Source: CAD feature listing. Evaluate the final solid. Frame: model axes, mm. Face numbers are marked on the shaded views. A direction names the side the tool comes from. Coordinates: 2 decimals unless noted, no trailing zeros. Write each loop counter-clockwise with the first axis right and the second up, starting at its lowest first coordinate (ties: lowest second). Pieces come first, ordered by that corner, then holes. Notation, with made-up numbers: (-28.75, 43) -> (5.25, 43) arc R22 ccw to (5.25, 62) -> close; hole circle Ø6 at (-7.5, 67). An arc over 180 degrees is marked (long way). Write item = value, one per line.
from build123d import *

# Parameters (mm, degrees)
SKETCH003_W  = 130
SKETCH003_H  = 30
PAD003_DEPTH = 150
SKETCH002_W  = 180
SKETCH002_H  = 65
PAD002_DEPTH = 145


with BuildPart() as body002:
    # Sketch003 → Pad003 (new body)
    with BuildSketch(Plane.XZ):
        with Locations((13.539826, -11.184382)):
            Rectangle(SKETCH003_W, SKETCH003_H)
    extrude(amount=PAD003_DEPTH)


with BuildPart() as body002_1:
    # Body002 placement: moved
    add(body002.part.moved(Location((0, 2, 0))))


with BuildPart() as cut:
    # Sketch002 → Pad002 (new body)
    with BuildSketch(Plane.XZ):
        Rectangle(SKETCH002_W, SKETCH002_H)
    extrude(amount=PAD002_DEPTH)

    # Cut: cut Body002
    add(body002_1.part, mode=Mode.SUBTRACT)


with BuildPart() as cut_1:
    # Cut placement: moved
    add(cut.part.moved(Location((0, 1, 0))))


solid = cut_1.part
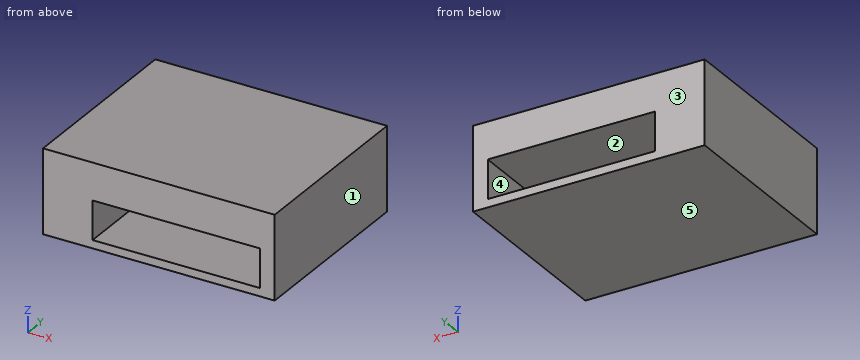
1) Cut plane C-C, the plane y = -60.5. Output: boundary loops of the cut face in (x, z).
Answer block:
outline = (-90, -32.5) -> (90, -32.5) -> (90, 32.5) -> (-90, 32.5) -> close; hole (-51.46, -26.18) -> (78.54, -26.18) -> (78.54, 3.82) -> (-51.46, 3.82) -> close
2) Cut plane A-A, the plane z = -4. Output: boundary loops of the cut face in (x, y), and give its area (3 significant figures).
Answer block:
outline = (-90, -144) -> (-51.46, -144) -> (-51.46, 1) -> (-90, 1) -> close; (78.54, -144) -> (90, -144) -> (90, 1) -> (78.54, 1) -> close
area = 7,250 mm2
3) Cut plane B-B, the plane x = -2. Output: boundary loops of the cut face in (y, z).
Answer block:
outline = (-144, -32.5) -> (1, -32.5) -> (1, -26.18) -> (-144, -26.18) -> close; (-144, 3.82) -> (1, 3.82) -> (1, 32.5) -> (-144, 32.5) -> close
4) Pull-direction query (Z, two-part tool) for the marked faces 3, 4 and 5; classes: +Z half, -Z half, draft (parallel to the pull), parting line (faces both ways), or undercut.
Answer block:
face_3 = draft
face_4 = undercut
face_5 = -Z half
5) First-contact query: pin 1 Ø12 at (x, z) = (-14.5, -25.5) entering from +Y. Flat tip, straight axial feed; report the tip coordinate or a pass-through.
Answer block:
pin_1 = 1
6) Material intervals for probe 1 along X at (y, z) = (-85.5, 1); probe 2 along Z at (x, y) = (-22, -97), sorted ascending. Write a range as [from, to].
Answer block:
probe_1 = [-90, -51.46], [78.54, 90]
probe_2 = [-32.5, -26.18], [3.82, 32.5]
7) Reachability of the marked faces 1 and 2 from +Z, -Z, +X, -X, +Y, -Y: full face, straight path, thin tool, end or side. Return the list, or none.
Answer block:
face_1 = +Z, -Z, +X, +Y, -Y
face_2 = +Y, -Y
